Autodesk Fusion 360 part; units mm, degrees
sketch "Skizze1" plane through (0, 0, 0) normal (0, 0, 1) x (1, 0, 0)
  line L0 (0, 118.8766) -> (0, -120.4869) construction
  line L1 (5, -90) -> (-5, -90)
  line L2 (-5, -90) -> (-5, 90)
  line L3 (-5, 90) -> (5, 90)
  line L4 (5, 90) -> (5, -90)
  line L5 (5, -90) -> (-5, 90) construction
  line L6 (-5, -90) -> (5, 90) construction
  circle A0 centre (0, 37.5) radius 1.25
  circle A1 centre (0, -37.5) radius 1.25
  circle A2 centre (0, 15) radius 1.75
  circle A3 centre (0, -15) radius 1.75
  circle A4 centre (0, 60) radius 1.75
  circle A5 centre (0, -60) radius 1.75
  line L7 (-5, 30) -> (5, 30)
  line L8 (-5, -30) -> (5, -30)
  line L9 (-5, -45) -> (5, -45)
  line L10 (-5, 45) -> (5, 45)
  line L11 (1.2702, -39.7) -> (2.5403, -37.5)
  line L12 (2.5403, -37.5) -> (1.2702, -35.3)
  line L13 (1.2702, -35.3) -> (-1.2702, -35.3)
  line L14 (-1.2702, -35.3) -> (-2.5403, -37.5)
  line L15 (-2.5403, -37.5) -> (-1.2702, -39.7)
  line L16 (-1.2702, -39.7) -> (1.2702, -39.7)
  line L17 (1.2702, 35.3) -> (2.5403, 37.5)
  line L18 (2.5403, 37.5) -> (1.2702, 39.7)
  line L19 (1.2702, 39.7) -> (-1.2702, 39.7)
  line L20 (-1.2702, 39.7) -> (-2.5403, 37.5)
  line L21 (-2.5403, 37.5) -> (-1.2702, 35.3)
  line L22 (-1.2702, 35.3) -> (1.2702, 35.3)
  circle A6 centre (0, 82.5) radius 1.25
  circle A7 centre (0, -82.5) radius 1.25
  line L23 (1.2702, 80.3) -> (2.5403, 82.5)
  line L24 (2.5403, 82.5) -> (1.2702, 84.7)
  line L25 (1.2702, 84.7) -> (-1.2702, 84.7)
  line L26 (-1.2702, 84.7) -> (-2.5403, 82.5)
  line L27 (-2.5403, 82.5) -> (-1.2702, 80.3)
  line L28 (-1.2702, 80.3) -> (1.2702, 80.3)
  line L29 (1.2702, -84.7) -> (2.5403, -82.5)
  line L30 (2.5403, -82.5) -> (1.2702, -80.3)
  line L31 (1.2702, -80.3) -> (-1.2702, -80.3)
  line L32 (-1.2702, -80.3) -> (-2.5403, -82.5)
  line L33 (-2.5403, -82.5) -> (-1.2702, -84.7)
  line L34 (-1.2702, -84.7) -> (1.2702, -84.7)
  line L35 (-5, -75) -> (5, -75)
  line L36 (-5, 75) -> (5, 75)
  point P0 (0, -37.5)
  point P1 (0, 37.5)
  point P2 (0, 82.5)
  point P3 (0, -82.5)
  dimension "d1" = 10
  dimension "d2" = 180
  dimension "d3" = 37.5
  dimension "d4" = 37.5
  dimension "d5" = 2.5
  dimension "d7" = 2.5
  dimension "d8" = 3.5
  dimension "d9" = 3.5
  dimension "d10" = 15
  dimension "d11" = 15
  dimension "d12" = 3.5
  dimension "d13" = 3.5
  dimension "d14" = 45
  dimension "d15" = 45
  dimension "d16" = 7.5
  dimension "d17" = 7.5
  dimension "d20" = 4.4
  dimension "d21" = 4.4
  dimension "d33" = 2.5
  dimension "d34" = 2.5
  dimension "d35" = 4.4
  dimension "d36" = 4.4
  dimension "d37" = 45
  dimension "d38" = 45
  dimension "d39" = 7.5
  dimension "d40" = 7.5
  dimension "d41" = 7.5
  dimension "d42" = 7.5
  dimension "d43" = 7.5
extrude "Extrusion1" add sketch "Skizze1" along normal blind 3 contours L1 L2 L4 L35 | L2 L4 L9 L35 | L2 L4 L8 L9 | L2 L4 L7 L8 | L2 L4 L7 L10 | L2 L4 L10 L36 | L2 L3 L4 L36 | L11 L12 L13 L14 L15 L16 | L17 L18 L19 L20 L21 L22 | L23 L24 L25 L26 L27 L28 | L29 L30 L31 L32 L33 L34
extrude "Extrusion2" add sketch "Skizze1" along normal blind 13 contours L1 L2 L4 L35 | L2 L4 L8 L9 | L2 L4 L7 L10 | L2 L3 L4 L36 | L11 L12 L13 L14 L15 L16 | L17 L18 L19 L20 L21 L22 | L23 L24 L25 L26 L27 L28 | L29 L30 L31 L32 L33 L34
extrude "Extrusion3" cut sketch "Skizze1" along normal blind 11 contours L11 L12 L13 L14 L15 L16 | L17 L18 L19 L20 L21 L22 | L23 L24 L25 L26 L27 L28 | L29 L30 L31 L32 L33 L34
extrude "Extrusion4" add sketch "Skizze1" along normal blind 9.2 contours L11 L12 L13 L14 L15 L16 | L17 L18 L19 L20 L21 L22 | L23 L24 L25 L26 L27 L28 | L29 L30 L31 L32 L33 L34
equation "d3 = ( 75 / 2 ) * 1 mm"
equation "d4 = ( 75 / 2 ) * 1 mm"
Model file for the job. Use its own axes, mm. A direction names the side the tool comes from. Give positions to 0.01 mm unless a question says otherwise; leave off trailing zeros. Order: outer loops, then holes, each group sorted by start corner. A loop starts at its lowest first (then second) coordinate and runs counter-clockwise, first axis right, second up. Notation, with made-up numbers: (80, 31.25) - (114, 31.25) arc R10 cw to (114, 35.25) - close; hole circle Ø2 at (-27.75, -12). An arc over 180 degrees is marked (long way). Return JSON: item names as keys, results as strings.
1) Flat gauge pins, fed straight in: P1, Ø3, axis at x = -1, y = -53, coming from the +Z side; P2, Ø3, axis at x = 0, y = -60, coming from the +Z side; P3, Ø5, axis at x = 1, y = 65.5, coming from the -Z side. Where does each tip first touch, or does it go through?
Geometry says:
{"P1": "z = 3", "P2": "through", "P3": "z = 0"}
2) Probe line 1 (Y direction, x = -3, z = 7.25); line 2 (X direction, y = -82.5, z = 11.85); line 3 (Z direction, x = -4, y = -23). List the from-to ranges inside material, lowest first. Write a range as from..to.
Geometry says:
{"line 1": "-90..-75, -45..-30, 30..45, 75..90", "line 2": "-5..-1.25, 1.25..5", "line 3": "0..3"}
3) Pull direction Y, two halves, no side cores. Call faces 1 (the flat face through (0, 90, 6)), 2 (the flat face through (1, -81, 9.2)), 3 (the flat face through (-5, -1, 2)): pulls with the +Y half, pulls with the -Y half, needs draft (parallel to the pull), parting line crosses it, or undercut.
Geometry says:
{"face 1": "pulls with the +Y half", "face 2": "undercut", "face 3": "needs draft"}
4) 3-axis set-ups, long thin cutter, end or side, ignore diameter. For faces 4 (the flat face through (1, -81, 11)), 5 (the flat face through (0, 1, 0)), 6 (the flat face through (2, -60, 3)): which of +Z, -Z, +X, -X, +Y, -Y reach the whole face in a straight line?
Geometry says:
{"face 4": "none", "face 5": "-Z, +X, -X, +Y, -Y", "face 6": "+Z, +X, -X"}
5) Cut at A-A, the plane y = 60. Give the cut face in (x, z), plus the area to 3 significant figures.
Geometry says:
{"outline": "(-5, 0) - (-1.75, 0) - (-1.75, 3) - (-5, 3) - close; (1.75, 0) - (5, 0) - (5, 3) - (1.75, 3) - close", "area": "19.5 mm²"}
6) Cut at B-B, the plane y = -20.5. Give the cut face in (x, z), plus the area to 3 significant figures.
Geometry says:
{"outline": "(-5, 0) - (5, 0) - (5, 3) - (-5, 3) - close", "area": "30.0 mm²"}
